from build123d import *

# Parameters (mm, degrees)
BOSS_EXTRUDE1_DEPTH     = 10
SKETCH3_R               = 1.5
CUT_EXTRUDE1_DEPTH      = 1
CUT_EXTRUDE1_DEPTH_BACK = 10


with BuildPart() as part:
    # Sketch1 → Boss-Extrude1 (new body)
    with BuildSketch(Plane.XY):
        Polygon((-1.5, -0.5), (0, -0.5), (1.5, -0.5), (1.5, -12.5), (4.5, -12.5), (4.5, 12.5), (-4.5, 12.5), (-4.5, -12.5), (-1.5, -12.5), align=None)
        with BuildLine():
            ThreePointArc((3, 7), (2.121320344, 4.878679656), (0, 4))
            ThreePointArc((0, 4), (-2.121320344, 9.121320344), (3, 7))
        make_face(mode=Mode.SUBTRACT)
    extrude(amount=BOSS_EXTRUDE1_DEPTH)

    # Sketch3 → Cut-Extrude1 (cut, two sides)
    with BuildSketch(Plane(origin=(4.5, 0, 0), x_dir=(0, 0, -1), z_dir=(1, 0, 0))) as cut_extrude1_sk:
        with Locations((-5, -5)):
            Circle(SKETCH3_R)
    extrude(amount=CUT_EXTRUDE1_DEPTH, mode=Mode.SUBTRACT)
    extrude(cut_extrude1_sk.sketch, amount=-CUT_EXTRUDE1_DEPTH_BACK, mode=Mode.SUBTRACT)


solid = part.part
Input: part model. Units: mm. Frame: model coordinates. A direction names the side the tool comes from. Give positions to 0.01 mm unless a question says otherwise; leave off trailing zeros. Write each loop counter-clockwise with the first axis right and the second up, starting at its lowest first coordinate (ties: lowest second). Pieces come first, ordered by that corner, then holes.
Q1. Section D-D, the plane z = 2.5. Output: boundary loops of the cut face in (x, y), plus the area to 3 significant figures.
Q2. Section A-A, the plane z = 5. Output: boundary loops of the cut face in (x, y), plus the area to 3 significant figures.
Q3. Set-up query: faces 4 (the face through (0, -0.5, 5)), 5 (the face through (3, -12.5, 5)). Return all of +Z, -Z, +X, -X, +Y, -Y with unobstructed straight access to the full face (end or side cutting, diameter ignored); none if empty.
Q4. Pull-direction query (Y, two-part tool) for faces 1 (the face through (-2.98, -3.99, 6.11)), 2 (the face through (-4.5, 0, 5)), 3 (the face through (-3, -12.5, 5)); classes: pulls with the +Y half, pulls with the -Y half, needs draft (parallel to the pull), parting line crosses it, or undercut.
Q5. Section C-C, the plane x = 2. Output: boundary loops of the cut face in (y, z), plus the area to 3 significant figures.
Q6. First-contact query: P1, Ø2.5, axis at y = -5, z = 5, coming from the +X side; P2, Ø1.5, axis at x = -0.5, z = 7, coming from the -Y side. Flat tips, straight axial feed; report the tip coordinate or a pass-through.
Q7. Section B-B, the plane y = -7. Output: boundary loops of the cut face in (x, z), plus the area to 3 significant figures.
Q8. Material intervals for probe 1 along Y at (x, z) = (3.45, 5); probe 2 along X at (y, z) = (-5.5, 8.25); probe 3 along Y at (x, z) = (0, 5), sorted ascending.
Filled in:
1. outline: (-4.5, -12.5) - (-1.5, -12.5) - (-1.5, -0.5) - (1.5, -0.5) - (1.5, -12.5) - (4.5, -12.5) - (4.5, 12.5) - (-4.5, 12.5) - close; hole circle Ø6 at (0, 7)
1. area: 161 mm2
2. outline: (-4.5, -12.5) - (-1.5, -12.5) - (-1.5, -6.5) - (-4.5, -6.5) - close; (-4.5, -3.5) - (-1.5, -3.5) - (-1.5, -0.5) - (1.5, -0.5) - (1.5, -3.5) - (4.5, -3.5) - (4.5, 12.5) - (-4.5, 12.5) - close; (1.5, -12.5) - (4.5, -12.5) - (4.5, -6.5) - (1.5, -6.5) - close; hole circle Ø6 at (0, 7)
2. area: 143 mm2
3. face 4: +Z, -Z, -Y
3. face 5: +Z, -Z, +X, -X, -Y
4. face 1: undercut
4. face 2: needs draft
4. face 3: pulls with the -Y half
5. outline: (-12.5, 0) - (4.76, 0) - (4.76, 10) - (-12.5, 10) - close; (9.24, 0) - (12.5, 0) - (12.5, 10) - (9.24, 10) - close; hole circle Ø3 at (-5, 5)
5. area: 198 mm2
6. P1: passes through
6. P2: stops at y = -0.5
7. outline: (-4.5, 0) - (-1.5, 0) - (-1.5, 10) - (-4.5, 10) - close; (1.5, 0) - (4.5, 0) - (4.5, 10) - (1.5, 10) - close
7. area: 60.0 mm2
8. probe 1: y = -12.5 to -6.5, -3.5 to 12.5
8. probe 2: x = -4.5 to -1.5, 1.5 to 4.5
8. probe 3: y = -0.5 to 4, 10 to 12.5
